```python
from build123d import *

# Parameters (mm, degrees)
SKETCH1_R           = 2.946896199
BOSS_EXTRUDE1_DEPTH = 1.5
SKETCH2_R           = 1.15
CUT_EXTRUDE1_DEPTH  = 12.783569069
SKETCH3_R           = 5.446896199
SKETCH3_R_2         = 2.946896199
BOSS_EXTRUDE2_DEPTH = 7
SKETCH4_R           = 4.25
BOSS_EXTRUDE3_DEPTH = 3
FILLET1_R           = 4
FILLET2_R           = 0.5
FILLET3_R           = 0.2


with BuildPart() as part:
    # Sketch1 → Boss-Extrude1 (new body)
    with BuildSketch(Plane(origin=(0, 0, 0), x_dir=(1, 0, 0), z_dir=(0, 1, 0))):
        with BuildLine():
            ThreePointArc((-4.282383784, -4.273603764), (0, -6.05), (4.282383784, -4.273603764))
            ThreePointArc((4.282383784, -4.273603764), (5.414251665, -3.516053121), (6.75, -3.25))
            ThreePointArc((6.75, -3.25), (10, 0), (6.75, 3.25))
            ThreePointArc((6.75, 3.25), (5.414251665, 3.516053121), (4.282383784, 4.273603764))
            ThreePointArc((4.282383784, 4.273603764), (0, 6.05), (-4.282383784, 4.273603764))
            ThreePointArc((-4.282383784, 4.273603764), (-5.414251665, 3.516053121), (-6.75, 3.25))
            ThreePointArc((-6.75, 3.25), (-10, 0), (-6.75, -3.25))
            ThreePointArc((-6.75, -3.25), (-5.414251665, -3.516053121), (-4.282383784, -4.273603764))
        make_face()
        with Locations(Location((0, 0, 0), (0, 0, 270))):
            Circle(SKETCH1_R, mode=Mode.SUBTRACT)
    extrude(amount=BOSS_EXTRUDE1_DEPTH)

    # Sketch2 → Cut-Extrude1 (cut, through all)
    with BuildSketch(Plane(origin=(0, 1.5, 0), x_dir=(1, 0, 0), z_dir=(0, 1, 0))):
        with Locations(Location((-6.75, 0, 0), (0, 0, 270))):
            Circle(SKETCH2_R)
        with Locations(Location((6.75, 0, 0), (0, 0, 90))):
            Circle(SKETCH2_R)
    extrude(amount=-CUT_EXTRUDE1_DEPTH, mode=Mode.SUBTRACT)

    # Sketch3 → Boss-Extrude2 (add)
    with BuildSketch(Plane(origin=(0, 1.5, 0), x_dir=(1, 0, 0), z_dir=(0, 1, 0))):
        with Locations(Location((0, 0, 0), (0, 0, 270))):
            Circle(SKETCH3_R)
        with Locations(Location((0, 0, 0), (0, 0, 270))):
            Circle(SKETCH3_R_2, mode=Mode.SUBTRACT)
    extrude(amount=BOSS_EXTRUDE2_DEPTH)

    # Sketch4 → Boss-Extrude3 (add)
    with BuildSketch(Plane(origin=(0, 8.5, 0), x_dir=(1, 0, 0), z_dir=(0, 1, 0))):
        with Locations(Location((0, 0, 0), (0, 0, 270))):
            Circle(SKETCH4_R)
    extrude(amount=BOSS_EXTRUDE3_DEPTH)

    # Fillet1
    # the kernel refuses this fillet: 4 mm, written as the material it takes off along each edge
    with BuildSketch(Plane(origin=(0, 11.5, 0), x_dir=(0, 0, 1), z_dir=(-1, 0, 0))) as fillet1_piece_1:
        with BuildLine():
            CenterArc((0.377016654, -4), FILLET1_R, 14.477512186, 75.522487814)
            Line((0.377016654, 0), (0.377016654, 0.08))
            Line((0.377016654, 0.08), (4.25, 0.08))
            Line((4.25, 0.08), (4.33, 0))
            ThreePointArc((4.33, 0), (4.33, -1.5), (4.327459667, -2.98))
            Line((4.327459667, -2.98), (4.25, -3))
        make_face()
    revolve(axis=Axis((0, 11.5, 0), (0, 1, 0)), mode=Mode.SUBTRACT)

    # Fillet2
    fillet2_edges = [part.edges().sort_by_distance(p)[0] for p in [
        (0, 8.5, -5.446896199),
    ]]
    fillet(fillet2_edges, radius=FILLET2_R)

    # Fillet3
    fillet3_edges = [part.edges().sort_by_distance(p)[0] for p in [
        (0, 1.5, -5.446896199),
    ]]
    fillet(fillet3_edges, radius=FILLET3_R)


solid = part.part
```
The listing builds one solid part. Answer for the finished solid, in the listing's coordinates (mm). A direction names the side the tool comes from. Give positions to 0.01 mm unless a question says otherwise; leave off trailing zeros. Order: outer loops, then holes, each group sorted by start corner. A loop starts at its lowest first (then second) coordinate and runs counter-clockwise, first axis right, second up. Notation, with made-up numbers: (57, 80) -> (71, 80) arc R19 cw to (71, 113) -> close; hole circle Ø6 at (5, -6). An arc over 180 degrees is marked (long way). Answer as a JSON object with one key per item and string values. Group by question number.
Item 1: Determine the mould class of faces 1 (the cylindrical face through (5.61, 0.76, 0.15)), 2 (the cylindrical face through (0.07, 0.74, -6.05)), 3 (the cylindrical face through (-0.07, 0.74, 6.05)) for opening direction Z: pulls with the +Z half, pulls with the -Z half, needs draft (parallel to the pull), parting line crosses it, or undercut.
Item 2: Flat-ended cylindrical pins translate along their axes: pin 1 (3.5 mm diameter, centred on x = -6.75, z = 0, fed in from +Y); pin 2 (4 mm diameter, centred on x = -1.5, y = 5, fed in from +Z); pin 3 (5 mm diameter, centred on y = 9, z = -0.5, fed in from +X); pin 4 (4 mm diameter, centred on x = 7.5, z = 3.5, fed in from -Y). Find the tip coordinate at first contact, or state that the pin passes through.
Item 3: The part is cut by section B-B on y = 3.75. Write down the section's boundary in (x, z).
Item 4: A tool of negligible diameter and unlimited length cuts with its end or side. For faces 4 (the cylindrical face through (10, 1, 0)), 5 (the flat face through (0, 8.5, 0)), 6 (the cylindrical face through (1.636, 4.801, 5.195)), from which of +Z, -Z, +X, -X, +Y, -Y can it reach the whole face along a straight path? Write none if from no direction.
Item 5: The part is cut by section C-C on z = 0. Give the number of separate pieces and of enclosed holes in the cut face, and give its area (3 significant figures).
Item 6: The part is cut by section A-A on x = 7. Write down the section's boundary in (y, z).
Item 7: Consider L1, parallel to X at y = 1.1, z = 0; L2, parallel to X at y = 2, z = 0; L3, parallel to Z at x = -6.75, y = 1.1. Determine where each line is inside the solid, lowest interval first. Write a range as from..to.
Result set:
{
 "1": {"face 1": "undercut", "face 2": "pulls with the -Z half", "face 3": "pulls with the +Z half"},
 "2": {"pin 1": "y = 8.5", "pin 2": "z = 5.45", "pin 3": "x = 5.45", "pin 4": "y = 0"},
 "3": {"outline": "circle Ø10.89 at (0, 0); hole circle Ø5.89 at (0, 0)"},
 "4": {"face 4": "+X, +Y, -Y", "face 5": "-Y", "face 6": "+Y"},
 "5": {"separate pieces": "3", "enclosed holes": "0", "area": "68.6 mm²"},
 "6": {"outline": "(0, -3.24) -> (1.5, -3.24) -> (1.5, -1.12) -> (0, -1.12) -> close; (0, 1.12) -> (1.5, 1.12) -> (1.5, 3.24) -> (0, 3.24) -> close"},
 "7": {"L1": "-10..-7.9, -5.6..-2.95, 2.95..5.6, 7.9..10", "L2": "-5.45..-2.95, 2.95..5.45", "L3": "-3.25..-1.15, 1.15..3.25"}
}
